```python
from build123d import *

# Parameters (mm, degrees)
SKETCH1_R           = 6.3627
SKETCH1_R_2         = 1.78435
BOSS_EXTRUDE1_DEPTH = 2.286


with BuildPart() as part:
    # Sketch1 → Boss-Extrude1 (new body)
    with BuildSketch(Plane.XZ):
        with BuildLine():
            Line((15.875, -19.05), (15.875, 19.05))
            ThreePointArc((15.875, 19.05), (0, 34.925), (-15.875, 19.05))
            Line((-15.875, 19.05), (-15.875, -19.05))
            ThreePointArc((-15.875, -19.05), (0, -34.925), (15.875, -19.05))
        make_face()
        with Locations(Location((0, -19.05, 0), (0, 0, 90))):
            Circle(SKETCH1_R, mode=Mode.SUBTRACT)
        with Locations(Location((0, 19.05, 0), (0, 0, 90))):
            Circle(SKETCH1_R, mode=Mode.SUBTRACT)
        with Locations(Location((9.779, 19.05, 0), (0, 0, 90))):
            Circle(SKETCH1_R_2, mode=Mode.SUBTRACT)
        with Locations(Location((6.914797213, 12.135202787, 0), (0, 0, 90))):
            Circle(SKETCH1_R_2, mode=Mode.SUBTRACT)
        with Locations(Location((0, 9.271, 0), (0, 0, 90))):
            Circle(SKETCH1_R_2, mode=Mode.SUBTRACT)
        with Locations(Location((-6.914797213, 12.135202787, 0), (0, 0, 90))):
            Circle(SKETCH1_R_2, mode=Mode.SUBTRACT)
        with Locations(Location((-9.779, 19.05, 0), (0, 0, 90))):
            Circle(SKETCH1_R_2, mode=Mode.SUBTRACT)
        with Locations(Location((-6.914797213, 25.964797213, 0), (0, 0, 90))):
            Circle(SKETCH1_R_2, mode=Mode.SUBTRACT)
        with Locations(Location((0, 28.829, 0), (0, 0, 90))):
            Circle(SKETCH1_R_2, mode=Mode.SUBTRACT)
        with Locations(Location((6.914797213, 25.964797213, 0), (0, 0, 90))):
            Circle(SKETCH1_R_2, mode=Mode.SUBTRACT)
        with Locations(Location((9.779, -19.05, 0), (0, 0, 90))):
            Circle(SKETCH1_R_2, mode=Mode.SUBTRACT)
        with Locations(Location((6.914797213, -12.135202787, 0), (0, 0, 90))):
            Circle(SKETCH1_R_2, mode=Mode.SUBTRACT)
        with Locations(Location((0, -9.271, 0), (0, 0, 90))):
            Circle(SKETCH1_R_2, mode=Mode.SUBTRACT)
        with Locations(Location((-6.914797213, -12.135202787, 0), (0, 0, 90))):
            Circle(SKETCH1_R_2, mode=Mode.SUBTRACT)
        with Locations(Location((-9.779, -19.05, 0), (0, 0, 90))):
            Circle(SKETCH1_R_2, mode=Mode.SUBTRACT)
        with Locations(Location((-6.914797213, -25.964797213, 0), (0, 0, 90))):
            Circle(SKETCH1_R_2, mode=Mode.SUBTRACT)
        with Locations(Location((0, -28.829, 0), (0, 0, 90))):
            Circle(SKETCH1_R_2, mode=Mode.SUBTRACT)
        with Locations(Location((6.914797213, -25.964797213, 0), (0, 0, 90))):
            Circle(SKETCH1_R_2, mode=Mode.SUBTRACT)
    extrude(amount=-BOSS_EXTRUDE1_DEPTH)


solid = part.part
```
Work out the finished part from the listing and answer in its coordinate system (mm). Round coordinates to 2 decimals unless told otherwise and drop trailing zeros. Loops run counter-clockwise (first coordinate to the right, second up) from the corner with the lowest first, then second, coordinate; pieces in that order, holes last. Notation, with made-up numbers: M -10.75,24 L 7.25,24 A24 ccw 7.25,36 Z; hole C 26.25,87 d1. An arc over 180 degrees is marked long. One line per question, with ' | ' between items.
Q1. Find section B-B, the plane z = -8.5. Give the vertices of the cut face in (x, y) (3 decimals), then the cut area to 3 significant figures.
Conclusion:
outline: M -15.875,0 L -1.609,0 L -1.609,2.286 L -15.875,2.286 Z; M 1.609,0 L 15.875,0 L 15.875,2.286 L 1.609,2.286 Z | area: 65.2 mm2
Q2. Consider line 1 along Z through (x, y) = (5, 1.7); line 2 along X through (y, z) = (1.55, -27); line 3 along X through (y, z) = (1.1, 20). Determine where each line is inside the solid, lowest interval first. Write a range as from..to.
Conclusion:
line 1: z = -34.12..-22.98, -15.12..15.12, 22.98..34.12 | line 2: x = -13.74..-8.37, -5.46..5.46, 8.37..13.74 | line 3: x = -15.85..-11.29, -8.27..-6.29, 6.29..8.27, 11.29..15.85
Q3. Find section C-C, the plane y = 0.9. State how many separate pieces and enclosed holes the cut face has, then the cut area to 3 significant figures.
Conclusion:
separate pieces: 1 | enclosed holes: 18 | area: 1,590 mm2
Q4. The mould has two halves that part along Z. Classify faces 1 (the flat face through (15.875, 1, 0)), 2 (the cylindrical face through (6.379, 1.127, -10.433)), 3 (the cylindrical face through (0.35, 1.13, 34.92)): +Z half, -Z half, draft (parallel to the pull), parting line (faces both ways), or undercut.
Conclusion:
face 1: draft | face 2: undercut | face 3: +Z half
Q5. This flat-tipped pin is pushed along its axis until it touches: pin 1 Ø4.5 at (x, z) = (-6.91, 25.96) entering from +Y. Where does it stop, or does it pass through?
Conclusion:
pin 1: stops at y = 2.29
Q6. Find section A-A, the plane x = 0. Give the vertices of the cut face in (y, z) (3 decimals).
Conclusion:
outline: M 0,-34.925 L 2.286,-34.925 L 2.286,-30.613 L 0,-30.613 Z; M 0,-27.045 L 2.286,-27.045 L 2.286,-25.413 L 0,-25.413 Z; M 0,-12.687 L 2.286,-12.687 L 2.286,-11.055 L 0,-11.055 Z; M 0,-7.487 L 2.286,-7.487 L 2.286,7.487 L 0,7.487 Z; M 0,11.055 L 2.286,11.055 L 2.286,12.687 L 0,12.687 Z; M 0,25.413 L 2.286,25.413 L 2.286,27.045 L 0,27.045 Z; M 0,30.613 L 2.286,30.613 L 2.286,34.925 L 0,34.925 Z
Q7. Find section D-D, the plane z = -23. Give the vertices of the cut face in (x, y).
Conclusion:
outline: M -15.38,0 L -4.99,0 L -4.99,2.29 L -15.38,2.29 Z; M 4.99,0 L 15.38,0 L 15.38,2.29 L 4.99,2.29 Z
